Geometry: final body of the model. Coordinates: model frame, mm. Face numbers are marked on the shaded views. Round coordinates to 2 decimals unless told otherwise and drop trailing zeros. Order: outer loops, then holes, each group sorted by start corner. A loop starts at its lowest first (then second) coordinate and runs counter-clockwise, first axis right, second up. Notation, with made-up numbers: (45.25, 46.25) -> (81.25, 46.25) arc R23 cw to (81.25, 67.25) -> close; hole circle Ø1 at (19.25, 32). An arc over 180 degrees is marked (long way). Put each result on its own line as item: value.
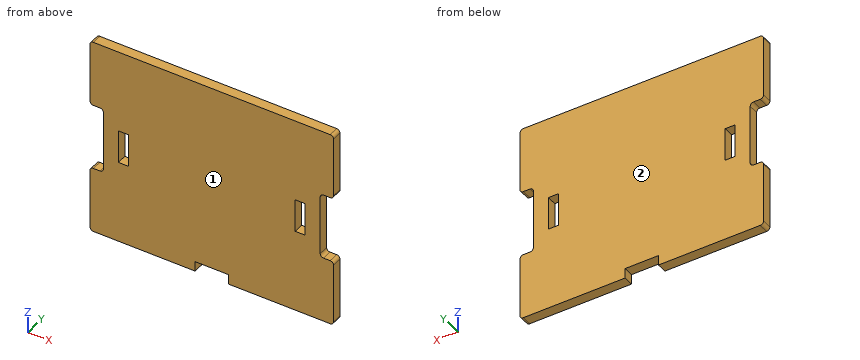
```python
from build123d import *

# Parameters (mm, degrees)
BOSS_EXTRUDE1_DEPTH     = 6
FILLET1_R               = 2
CUT_EXTRUDE1_DEPTH      = 95.683683917
CUT_EXTRUDE1_DEPTH_BACK = 95.683683917
SKETCH2_W               = 6
SKETCH2_H               = 20
SKETCH3_W               = 20
SKETCH3_H               = 6
CUT_EXTRUDE2_DEPTH      = 95.683683917


with BuildPart() as part:
    # Sketch1 → Boss-Extrude1 (new body)
    with BuildSketch(Plane(origin=(0, 0, 0), x_dir=(1, 0, 0), z_dir=(0, 1, 0))):
        Polygon((65, 20), (65, -20), (73, -20), (73, -60), (-73, -60), (-73, -20), (-65, -20), (-65, 20), (-73, 20), (-73, 60), (73, 60), (73, 20), align=None)
    extrude(amount=BOSS_EXTRUDE1_DEPTH)

    # Fillet1
    fillet1_edges = [part.edges().sort_by_distance(p)[0] for p in [
        (65, 3, 20),
        (73, 3, 20),
        (73, 3, 60),
        (-73, 3, 60),
        (-73, 3, 20),
        (-65, 3, 20),
        (-65, 3, -20),
        (-73, 3, -20),
        (-73, 3, -60),
        (73, 3, -60),
        (73, 3, -20),
        (65, 3, -20),
    ]]
    fillet(fillet1_edges, radius=FILLET1_R)

    # Sketch2 → Cut-Extrude1 (cut, two sides: drawn at the far end of the back side and taken through both)
    with BuildSketch(Plane(origin=(0, 6, 0), x_dir=(1, 0, 0), z_dir=(0, 1, 0)).offset(-CUT_EXTRUDE1_DEPTH_BACK)):
        with Locations((53, 0)):
            Rectangle(SKETCH2_W, SKETCH2_H)
        with Locations((-53, 0)):
            Rectangle(SKETCH2_W, SKETCH2_H)
    extrude(amount=CUT_EXTRUDE1_DEPTH + CUT_EXTRUDE1_DEPTH_BACK, mode=Mode.SUBTRACT)

    # Sketch3 → Cut-Extrude2 (cut, through all)
    with BuildSketch(Plane(origin=(0, 6, 0), x_dir=(1, 0, 0), z_dir=(0, 1, 0))):
        with Locations((0, 57)):
            Rectangle(SKETCH3_W, SKETCH3_H)
    extrude(amount=-CUT_EXTRUDE2_DEPTH, mode=Mode.SUBTRACT)


solid = part.part
```
1. Draft query along Y for the marked faces 1 and 2. Return one class per face: +Y half, -Y half, draft (parallel to the pull), parting line (faces both ways), or undercut.
Ans:
face 1: -Y half
face 2: +Y half
2. Contact query for flat-ended pins moving along their axis: P1, Ø1.8, axis at y = 2, z = -3, coming from the +X side; P2, Ø1, axis at y = 4, z = 21, coming from the -X side; P3, Ø3, axis at y = 3, z = 3, coming from the -X side. Output: stop coordinate, or through.
Ans:
P1: x = 65
P2: x = -72.94
P3: x = -65
3. Cut plane B-B on z = -6. Return loops of the section in (x, y), and give its area (3 significant figures).
Ans:
outline: (-65, 0) -> (-56, 0) -> (-56, 6) -> (-65, 6) -> close; (-50, 0) -> (50, 0) -> (50, 6) -> (-50, 6) -> close; (56, 0) -> (65, 0) -> (65, 6) -> (56, 6) -> close
area: 708 mm²
4. Cut plane C-C on y = 5.1. State how many separate pieces and enclosed holes the cut face has, and give its area (3 significant figures).
Ans:
separate pieces: 1
enclosed holes: 2
area: 16,500 mm²
5. Material intervals for probe 1 along X at (y, z) = (5.4, -1.5); probe 2 along X at (y, z) = (5.15, -17); probe 3 along Z at (x, y) = (-8.5, 5.4), sorted ascending.
Ans:
probe 1: -65 to -56, -50 to 50, 56 to 65
probe 2: -65 to 65
probe 3: -54 to 60
6. Cut plane A-A on x = 52.5. Return loops of the section in (y, z), and give its area (3 significant figures).
Ans:
outline: (0, -60) -> (6, -60) -> (6, -10) -> (0, -10) -> close; (0, 10) -> (6, 10) -> (6, 60) -> (0, 60) -> close
area: 600 mm²
